Source: CAD feature listing. Evaluate the final solid. Frame: model axes, mm. Round coordinates to 2 decimals unless told otherwise and drop trailing zeros. Order: outer loops, then holes, each group sorted by start corner. A loop starts at its lowest first (then second) coordinate and runs counter-clockwise, first axis right, second up. Notation, with made-up numbers: (-38.5, -24) -> (-30.5, -24) arc R10 ccw to (-30.5, -6) -> close; hole circle Ø6 at (85, 16). An arc over 180 degrees is marked (long way). Answer as CSV lines item,"result". Start each with the question number.
(1) Contact query for flat-ended pins moving along their axis: P1, Ø1, axis at x = -2, y = 23, coming from the +Z side; P2, Ø5, axis at y = 20, z = 3.5, coming from the -X side; P3, Ø1.5, axis at x = 3, y = 13.5, coming from the +Z side. Output: stop coordinate, or through.
(2) Line query: line 1 along Y through (x, z) = (-5.25, 0.75); line 2 along Z through (x, y) = (0, -3.5); line 3 along X through (y, z) = (8, 4.75). Output: solid intervals per line, ascending. Write a range as from..to.
(3) Section query A-A (y = 23). Output: boundary loops of the cut face in (x, z), plus the area to 3 significant figures.
```python
from build123d import *

# Parameters (mm, degrees)
CROQUIS1_R              = 6
SALIENTE_EXTRUIR1_DEPTH = 30
CROQUIS3_R              = 5
SALIENTE_EXTRUIR2_DEPTH = 1
CROQUIS4_R              = 6
SALIENTE_EXTRUIR3_DEPTH = 5
CROQUIS5_R              = 0.35
CORTAR_EXTRUIR1_DEPTH   = 5


with BuildPart() as part:
    # Croquis1 → Saliente-Extruir1 (new body)
    with BuildSketch(Plane(origin=(0, 0, 0), x_dir=(1, 0, 0), z_dir=(0, 1, 0))):
        Circle(CROQUIS1_R)
    extrude(amount=SALIENTE_EXTRUIR1_DEPTH)

    # Croquis3 → Saliente-Extruir2 (add)
    with BuildSketch(Plane.XZ):
        Circle(CROQUIS3_R)
    extrude(amount=SALIENTE_EXTRUIR2_DEPTH)

    # Croquis4 → Saliente-Extruir3 (add)
    with BuildSketch(Plane.XZ.offset(1)):
        Circle(CROQUIS4_R)
    extrude(amount=SALIENTE_EXTRUIR3_DEPTH)

    # Croquis5 → Cortar-Extruir1 (cut)
    with BuildSketch(Plane.XZ.offset(6)):
        with Locations((0, 6)):
            Circle(CROQUIS5_R)
        with Locations((1.247470145, 5.868885604)):
            Circle(CROQUIS5_R)
        with Locations((2.440419858, 5.481272746)):
            Circle(CROQUIS5_R)
        with Locations((3.526711514, 4.854101966)):
            Circle(CROQUIS5_R)
        with Locations((4.458868953, 4.014783638)):
            Circle(CROQUIS5_R)
        with Locations((5.196152423, 3)):
            Circle(CROQUIS5_R)
        with Locations((5.706339098, 1.854101966)):
            Circle(CROQUIS5_R)
        with Locations((5.967131372, 0.62717078)):
            Circle(CROQUIS5_R)
        with Locations((5.967131372, -0.62717078)):
            Circle(CROQUIS5_R)
        with Locations((5.706339098, -1.854101966)):
            Circle(CROQUIS5_R)
        with Locations((5.196152423, -3)):
            Circle(CROQUIS5_R)
        with Locations((4.458868953, -4.014783638)):
            Circle(CROQUIS5_R)
        with Locations((3.526711514, -4.854101966)):
            Circle(CROQUIS5_R)
        with Locations((2.440419858, -5.481272746)):
            Circle(CROQUIS5_R)
        with Locations((1.247470145, -5.868885604)):
            Circle(CROQUIS5_R)
        with Locations((0, -6)):
            Circle(CROQUIS5_R)
        with Locations((-1.247470145, -5.868885604)):
            Circle(CROQUIS5_R)
        with Locations((-2.440419858, -5.481272746)):
            Circle(CROQUIS5_R)
        with Locations((-3.526711514, -4.854101966)):
            Circle(CROQUIS5_R)
        with Locations((-4.458868953, -4.014783638)):
            Circle(CROQUIS5_R)
        with Locations((-5.196152423, -3)):
            Circle(CROQUIS5_R)
        with Locations((-5.706339098, -1.854101966)):
            Circle(CROQUIS5_R)
        with Locations((-5.967131372, -0.62717078)):
            Circle(CROQUIS5_R)
        with Locations((-5.967131372, 0.62717078)):
            Circle(CROQUIS5_R)
        with Locations((-5.706339098, 1.854101966)):
            Circle(CROQUIS5_R)
        with Locations((-5.196152423, 3)):
            Circle(CROQUIS5_R)
        with Locations((-4.458868953, 4.014783638)):
            Circle(CROQUIS5_R)
        with Locations((-3.526711514, 4.854101966)):
            Circle(CROQUIS5_R)
        with Locations((-2.440419858, 5.481272746)):
            Circle(CROQUIS5_R)
        with Locations((-1.247470145, 5.868885604)):
            Circle(CROQUIS5_R)
    extrude(amount=-CORTAR_EXTRUIR1_DEPTH, mode=Mode.SUBTRACT)


solid = part.part
```
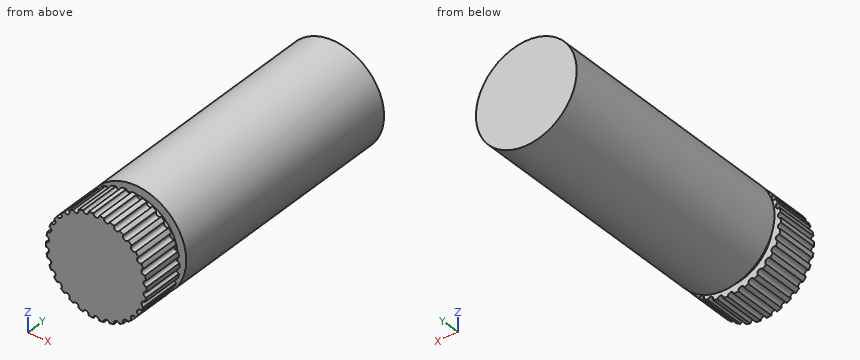
Answer block:
1,P1,"z = 5.81"
1,P2,"x = -5.92"
1,P3,"z = 5.56"
2,line 1,"-6..-1, 0..30"
2,line 2,"-5.65..5.65"
2,line 3,"-3.67..3.67"
3,outline,"circle Ø12 at (0, 0)"
3,area,"113 mm2"
